The listing builds one solid part. Answer for the finished solid, in the listing's coordinates (mm). A direction names the side the tool comes from. Coordinates: 2 decimals unless noted, no trailing zeros. Order: outer loops, then holes, each group sorted by start corner. A loop starts at its lowest first (then second) coordinate and runs counter-clockwise, first axis right, second up. Notation, with made-up numbers: (3, 52) -> (34, 52) arc R13 ccw to (34, 70) -> close; hole circle Ø7 at (21, -2.75). An arc over 180 degrees is marked (long way). Answer in a Markdown table with one row per item.
```python
from build123d import *

# Parameters (mm, degrees)
BOSS_EXTRUDE1_DEPTH = 3.15
CUT_EXTRUDE1_DEPTH  = 2.05
BOSS_EXTRUDE2_DEPTH = 2.05


with BuildPart() as part:
    # Sketch1 → Boss-Extrude1 (new body)
    with BuildSketch(Plane.XY):
        Polygon((0, 0), (14.25, 0), (14.25, 1.32), (1.32, 14.25), (0, 14.25), align=None)
    extrude(amount=-BOSS_EXTRUDE1_DEPTH)

    # Sketch2 → Cut-Extrude1 (cut)
    with BuildSketch(Plane(origin=(0, 0, -3.15), x_dir=(-1, 0, 0), z_dir=(0, 0, -1))):
        Polygon((-14.25, 1.32), (-1.32, 1.32), (-1.32, 14.25), align=None)
    extrude(amount=-CUT_EXTRUDE1_DEPTH, mode=Mode.SUBTRACT)

    # Sketch3 → Boss-Extrude2 (add)
    with BuildSketch(Plane(origin=(0, 0, -1.1), x_dir=(-1, 0, 0), z_dir=(0, 0, -1))):
        with BuildLine():
            Line((-10.0477417, 5.5222583), (-5.5222583, 10.0477417))
            ThreePointArc((-5.5222583, 10.0477417), (-5.5222583, 5.5222583), (-10.0477417, 5.5222583))
        make_face()
        with BuildLine():
            Line((-8.659427284, 5.496359153), (-5.496359153, 8.659427284))
            ThreePointArc((-5.496359153, 8.659427284), (-6.052588386, 6.052588386), (-8.659427284, 5.496359153))
        make_face(mode=Mode.SUBTRACT)
    extrude(amount=BOSS_EXTRUDE2_DEPTH)


solid = part.part
```
(1) A cutting plane is placed at B-B, the plane y = 4. Determine the outline of the cut face in (x, z), then the cut area to 3 significant figures.
Check values:
| item | result |
|---|---|
| outline | (0, -3.15) -> (1.32, -3.15) -> (1.32, -1.1) -> (11.57, -1.1) -> (11.57, 0) -> (0, 0) -> close |
| area | 15.4 mm² |
(2) A flat-ended cylindrical pin translates along its axis: pin 1 (1.6 mm diameter, centred on x = 8.5, z = -2.5, fed in from +Y). Find the tip coordinate at first contact, or state that the pin passes through.
Check values:
| item | result |
|---|---|
| pin 1 | y = 7.87 |
(3) Find the intervals of material crossed by line 1 along X through (y, z) = (6, -1.7); line 2 along Y through (x, z) = (6.5, -2.3), in increasing order. Write a range as from..to.
Check values:
| item | result |
|---|---|
| line 1 | 0..1.32, 5.13..6.11, 8.16..9.57 |
| line 2 | 0..1.32, 4.85..5.7, 7.66..9.07 |
(4) Which of the six approach directions +Z, -Z, +X, -X, +Y, -Y give full straight-line access (tool end or side, diameter ignored) to faces 4 (the flat face through (6.7, 6.7, -1.1)), 5 (the flat face through (1.32, 8, -2)), 6 (the flat face through (8, 7, -3.15)), 7 (the flat face through (8, 1.32, -2)), 8 (the flat face through (0, 7, -2))?
Check values:
| item | result |
|---|---|
| face 4 | -Z |
| face 5 | -Z, +Y |
| face 6 | -Z, +X, -X, +Y, -Y |
| face 7 | -Z, +X |
| face 8 | +Z, -Z, -X, +Y, -Y |
(5) For a pull along X with two mould halves and no side action, classify faces 1 (the flat face through (7.1, 7.056, -2.111)), 2 (the flat face through (7.88, 7.69, -1.2)), 3 (the flat face through (5, 6, 0)) as released by +X, released by -X, zero draft, split by the parting line, or undercut.
Check values:
| item | result |
|---|---|
| face 1 | undercut |
| face 2 | released by +X |
| face 3 | zero draft |
(6) A cutting plane is placed at A-A, the plane z = -2.05. Determine the outline of the cut face in (x, y) (3 decimals).
Check values:
| item | result |
|---|---|
| outline | (0, 0) -> (14.25, 0) -> (14.25, 1.32) -> (1.32, 1.32) -> (1.32, 14.25) -> (0, 14.25) -> close; (5.522, 10.048) arc R3.2 ccw to (10.048, 5.522) -> close; hole (5.496, 8.659) arc R2.45 ccw to (8.659, 5.496) -> close |
(7) A cutting plane is placed at C-C, the plane x = 13.5. Determine the outline of the cut face in (y, z), then the cut area to 3 significant figures.
Check values:
| item | result |
|---|---|
| outline | (0, -3.15) -> (1.32, -3.15) -> (1.32, -1.1) -> (2.07, -1.1) -> (2.07, 0) -> (0, 0) -> close |
| area | 4.98 mm² |
(8) A cutting plane is placed at D-D, the plane z = -0.9. Determine the outline of the cut face in (x, y), then the cut area to 3 significant figures.
Check values:
| item | result |
|---|---|
| outline | (0, 0) -> (14.25, 0) -> (14.25, 1.32) -> (1.32, 14.25) -> (0, 14.25) -> close |
| area | 119 mm² |
